Geometry: final body of the model. Coordinates: model frame, mm. Face numbers are marked on the shaded views. Coordinates: 2 decimals unless noted, no trailing zeros. Loops run counter-clockwise (first coordinate to the right, second up) from the corner with the lowest first, then second, coordinate; pieces in that order, holes last. Notation, with made-up numbers: (8, 60.25) - (65, 60.25) arc R28 ccw to (65, 85.25) - close; hole circle Ø10 at (29, 51). An arc over 180 degrees is marked (long way). Answer in a Markdown table with one row per item.
from build123d import *

# Parameters (mm, degrees)
SKETCH_1_W          = 250
SKETCH_1_H          = 39.5
EXTRUDE_1_DEPTH     = 2
SKETCH_2_R          = 2.5
SKETCH_2_R_2        = 1.5
EXTRUDE_2_DEPTH     = 3
FILLET_1_R          = 2.5
SKETCH_6_R          = 2.5
SKETCH_6_R_2        = 1.5
EXTRUDE_3_DEPTH     = 3
CUT_EXTRUDE_START   = -1
SKETCH_7_R          = 1.5
CUT_EXTRUDE_1_DEPTH = 1
SKETCH_8_R          = 1.5
CUT_EXTRUDE_2_DEPTH = 1
SKETCH_9_R          = 2.5
SKETCH_9_R_2        = 1.5
EXTRUDE_5_DEPTH     = 10.5
SKETCH_10_W         = 39.5
SKETCH_10_H         = 2
EXTRUDE_6_DEPTH     = 52
SKETCH_11_R         = 2.5
SKETCH_11_R_2       = 1.5
EXTRUDE_7_DEPTH     = 10.5
SKETCH_13_W         = 58
SKETCH_13_H         = 13.949858628
SKETCH_13_W_2       = 10.867061712
EXTRUDE_8_DEPTH     = 9
SKETCH_14_R         = 3
SKETCH_14_R_2       = 2
EXTRUDE_9_DEPTH     = 10.5


with BuildPart() as part:
    # 草图1 → 凸台-拉伸1 (new body)
    with BuildSketch(Plane(origin=(0, 0, 0), x_dir=(1, 0, 0), z_dir=(0, 1, 0))):
        with Locations((-84.429225121, -3.30093938)):
            Rectangle(SKETCH_1_W, SKETCH_1_H)
    extrude(amount=EXTRUDE_1_DEPTH)

    # 草图2 → 凸台-拉伸2 (add)
    with BuildSketch(Plane(origin=(0, 2, 0), x_dir=(1, 0, 0), z_dir=(0, 1, 0))):
        with Locations(Location((38.070774879, 13.94906062, 0), (0, 0, 90))):
            Circle(SKETCH_2_R)
        with Locations(Location((38.070774879, 13.94906062, 0), (0, 0, 270))):
            Circle(SKETCH_2_R_2, mode=Mode.SUBTRACT)
    extrude(amount=EXTRUDE_2_DEPTH)

    # 圆角1
    fillet_1_edges = [part.edges().sort_by_distance(p)[0] for p in [
        (40.570774879, 1, -16.44906062),
    ]]
    fillet(fillet_1_edges, radius=FILLET_1_R)

    # 草图6 → 凸台-拉伸3 (add)
    with BuildSketch(Plane(origin=(0, 2, 0), x_dir=(1, 0, 0), z_dir=(0, 1, 0))):
        with Locations(Location((-206.929225121, 13.94906062, 0), (0, 0, 90))):
            Circle(SKETCH_6_R)
        with Locations(Location((-206.929225121, 13.94906062, 0), (0, 0, 270))):
            Circle(SKETCH_6_R_2, mode=Mode.SUBTRACT)
    extrude(amount=EXTRUDE_3_DEPTH)

    # 草图7 → 切除-拉伸1 (cut)
    with BuildSketch(Plane(origin=(0, 2, 0), x_dir=(1, 0, 0), z_dir=(0, 1, 0)).offset(CUT_EXTRUDE_START)):
        with Locations(Location((38.070774879, 13.94906062, 0), (0, 0, 270))):
            Circle(SKETCH_7_R)
    extrude(amount=CUT_EXTRUDE_1_DEPTH, mode=Mode.SUBTRACT)

    # 草图8 → 切除-拉伸2 (cut)
    with BuildSketch(Plane(origin=(0, 2, 0), x_dir=(1, 0, 0), z_dir=(0, 1, 0)).offset(CUT_EXTRUDE_START)):
        with Locations(Location((-206.929225121, 13.94906062, 0), (0, 0, 270))):
            Circle(SKETCH_8_R)
    extrude(amount=CUT_EXTRUDE_2_DEPTH, mode=Mode.SUBTRACT)

    # 草图9 → 凸台-拉伸5 (add)
    # profile 1 of 2: a face of its own
    with BuildSketch(Plane(origin=(0, 2, 0), x_dir=(1, 0, 0), z_dir=(0, 1, 0))):
        with Locations(Location((23.570774879, -13.05093938, 0), (0, 0, 90))):
            Circle(SKETCH_9_R)
        with Locations(Location((23.570774879, -13.05093938, 0), (0, 0, 90))):
            Circle(SKETCH_9_R_2, mode=Mode.SUBTRACT)
    # profile 2 of 2: a face of its own
    with BuildSketch(Plane(origin=(0, 2, 0), x_dir=(1, 0, 0), z_dir=(0, 1, 0))):
        with Locations(Location((-34.429225121, -13.05093938, 0), (0, 0, 90))):
            Circle(SKETCH_9_R)
        with Locations(Location((-34.429225121, -13.05093938, 0), (0, 0, 90))):
            Circle(SKETCH_9_R_2, mode=Mode.SUBTRACT)
    extrude(amount=EXTRUDE_5_DEPTH)

    # 草图10 → 凸台-拉伸6 (add)
    with BuildSketch(Plane.ZY.offset(209.429225121)):
        with Locations((3.30093938, 1)):
            Rectangle(SKETCH_10_W, SKETCH_10_H)
    extrude(amount=EXTRUDE_6_DEPTH)

    # 草图11 → 凸台-拉伸7 (add)
    # profile 1 of 2: a face of its own
    with BuildSketch(Plane(origin=(0, 2, 0), x_dir=(1, 0, 0), z_dir=(0, 1, 0))):
        with Locations(Location((-252.299570288, -15.05093938, 0), (0, 0, 90))):
            Circle(SKETCH_11_R)
        with Locations(Location((-252.299570288, -15.05093938, 0), (0, 0, 90))):
            Circle(SKETCH_11_R_2, mode=Mode.SUBTRACT)
    # profile 2 of 2: a face of its own
    with BuildSketch(Plane(origin=(0, 2, 0), x_dir=(1, 0, 0), z_dir=(0, 1, 0))):
        with Locations(Location((-219.899570288, -15.05093938, 0), (0, 0, 90))):
            Circle(SKETCH_11_R)
        with Locations(Location((-219.899570288, -15.05093938, 0), (0, 0, 90))):
            Circle(SKETCH_11_R_2, mode=Mode.SUBTRACT)
    extrude(amount=EXTRUDE_7_DEPTH)

    # 草图13 → 凸台-拉伸8 (add)
    with BuildSketch(Plane(origin=(0, 2, 0), x_dir=(1, 0, 0), z_dir=(0, 1, 0))):
        with Locations((-5.429225121, -1.132807322)):
            Rectangle(SKETCH_13_W, SKETCH_13_H)
        with Locations((-234.073282944, -1.132807322)):
            Rectangle(SKETCH_13_W_2, SKETCH_13_H)
    extrude(amount=EXTRUDE_8_DEPTH)

    # 草图14 → 凸台-拉伸9 (add)
    # profile 1 of 2: a face of its own
    with BuildSketch(Plane(origin=(0, 2, 0), x_dir=(1, 0, 0), z_dir=(0, 1, 0))):
        with Locations(Location((-141.341724895, -13.05093938, 0), (0, 0, 90))):
            Circle(SKETCH_14_R)
        with Locations(Location((-141.341724895, -13.05093938, 0), (0, 0, 90))):
            Circle(SKETCH_14_R_2, mode=Mode.SUBTRACT)
    # profile 2 of 2: a face of its own
    with BuildSketch(Plane(origin=(0, 2, 0), x_dir=(1, 0, 0), z_dir=(0, 1, 0))):
        with Locations(Location((-157.341724895, -13.05093938, 0), (0, 0, 90))):
            Circle(SKETCH_14_R)
        with Locations(Location((-157.341724895, -13.05093938, 0), (0, 0, 90))):
            Circle(SKETCH_14_R_2, mode=Mode.SUBTRACT)
    extrude(amount=EXTRUDE_9_DEPTH)


solid = part.part
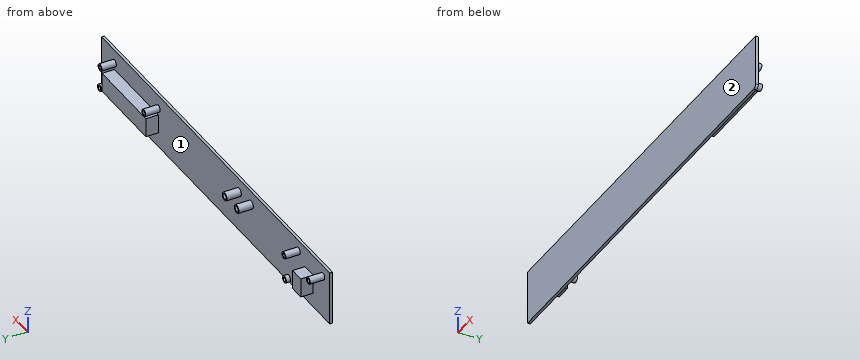
(1) Cut plane B-B on x = -8. Output: boundary loops of the cut face in (y, z).
Verdict:
| item | result |
|---|---|
| outline | (0, -16.45) - (2, -16.45) - (2, -5.84) - (11, -5.84) - (11, 8.11) - (2, 8.11) - (2, 23.05) - (0, 23.05) - close |
(2) Pull-direction query (X, two-part tool) for the marked faces 1 and 2; classes: pulls with the +X half, pulls with the -X half, needs draft (parallel to the pull), parting line crosses it, or undercut.
Verdict:
| item | result |
|---|---|
| face 1 | undercut |
| face 2 | needs draft |
(3) Ray query, probe 1 along X at (y, z) = (5.75, 0); probe 2 along Y at (x, z) = (-133, -9); probe 3 along Y at (x, z) = (-11, -3). Return the intervals inside material, ascending.
Verdict:
| item | result |
|---|---|
| probe 1 | x = -239.51 to -228.64, -34.43 to 23.57 |
| probe 2 | y = 0 to 2 |
| probe 3 | y = 0 to 11 |
(4) Cut plane D-D on x = -55. Output: boundary loops of the cut face in (y, z), then the cut area to 3 significant figures.
Verdict:
| item | result |
|---|---|
| outline | (0, -16.45) - (2, -16.45) - (2, 23.05) - (0, 23.05) - close |
| area | 79.0 mm² |
(5) Cut plane C-C on z = 5. Output: boundary loops of the cut face in (x, y), then the cut area to 3 significant figures.
Verdict:
| item | result |
|---|---|
| outline | (-261.43, 0) - (40.57, 0) - (40.57, 2) - (23.57, 2) - (23.57, 11) - (-34.43, 11) - (-34.43, 2) - (-228.64, 2) - (-228.64, 11) - (-239.51, 11) - (-239.51, 2) - (-261.43, 2) - close |
| area | 1,220 mm² |
(6) Cut plane A-A on y = 7.75. State how many separate pieces and enclosed holes the cut face has, then the cut area to 3 significant figures.
Verdict:
| item | result |
|---|---|
| separate pieces | 8 |
| enclosed holes | 6 |
| area | 1,040 mm² |
(7) First-contact query: pin 1 Ø4 at (x, z) = (7.5, -8) entering from +Y; pin 2 Ø11 at (x, z) = (-6.5, 3) entering from +Y; pin 3 Ø4.5 at (y, z) = (4.5, 0) entering from -X. Flat tips, straight axial feed; report the tip coordinate or a pass-through.
Verdict:
| item | result |
|---|---|
| pin 1 | stops at y = 2 |
| pin 2 | stops at y = 11 |
| pin 3 | stops at x = -239.51 |
